Geometry: final body of the model. Coordinates: model frame, mm. A direction names the side the tool comes from. Round coordinates to 2 decimals unless told otherwise and drop trailing zeros. Return JSON: item names as keys, results as strings. Group by question number.
1. Draft query along X for faces 1 (the face through (15, 20, 13.994)), 2 (the face through (22, 29, 11.613)), 3 (the face through (24.072, 37.706, 11.299)). Return one class per face: +X half, -X half, draft (parallel to the pull), parting line (faces both ways), or undercut.
2. Material intervals for probe 1 along Y at (x, z) = (18, 12); probe 2 along Y at (x, z) = (18.5, 12); probe 3 along Z at (x, y) = (14.5, 37), sorted ascending.
3. First-contact query: pin 1 Ø1.5 at (y, z) = (7.5, 11.5) entering from +X; pin 2 Ø3 at (x, z) = (26.5, 13) entering from -Y; pin 3 Ø5 at (y, z) = (15.5, 12.5) entering from -X. Flat tips, straight axial feed; report the tip coordinate or a pass-through.
4. Set-up query: faces 4 (the face through (18, 0, 11)), 5 (the face through (11.883, 10.519, 12.82)), 6 (the face through (25.615, 17.844, 7.981)). Return all of +Z, -Z, +X, -X, +Y, -Y with unobstructed straight access to the full face (end or side cutting, diameter ignored); none if empty.
from build123d import *

# Parameters (mm, degrees)
F1_ANGLE = 18.5
F2_R     = 7.9375
F3_DEPTH = 2.38125


with BuildPart() as f1:
    # F0 (on Front) → F1 (revolve)
    with BuildSketch(Plane.XZ):
        with BuildLine():
            Line((24.2297330525, 13.9939050769), (8.419544983, 13.9939050769))
            add(Edge.make_bspline(
                [(8.419544983, 13.9939050769), (8.3193296588, 12.729684062), (9.3964822164, 9.926852923), (14.9424578975, 8.5146570379), (21.1633145653, 6.8517774271), (23.2589200169, 4.9192732328), (24.1671312945, 4.0402704404)],
                knots=[0.4603012927, 0.4603012927, 0.4603012927, 0.4603012927, 0.5552126989, 0.6720441254, 0.8004871988, 0.8904119657, 0.8904119657, 0.8904119657, 0.8904119657], degree=3))
            Line((24.1671312945, 4.0402704404), (24.2297330525, 13.9939050769))
        make_face()
    revolve(axis=Axis((136.7642762608, 0, 8.3261267356), (0, 0, -1)), revolution_arc=F1_ANGLE)

    # F2 (on face) → F3 (cut)
    with BuildSketch(Plane.XY.offset(13.9939050769)):
        with Locations((22.9123420723, 28.597757378)):
            Circle(F2_R)
        with Locations((19.7691471926, 9.6189003033)):
            Circle(F2_R)
    extrude(amount=-F3_DEPTH, mode=Mode.SUBTRACT)


solid = f1.part
Taken from the geometry:
{
 "1": {"face 1": "draft", "face 2": "undercut", "face 3": "+X half"},
 "2": {"probe 1": "0 to 1.88, 17.36 to 22.36, 34.83 to 39.74", "probe 2": "0 to 1.78, 17.45 to 22, 35.2 to 39.57", "probe 3": "11.49 to 13.99"},
 "3": {"pin 1": "x = 24.52", "pin 2": "y = 15.33", "pin 3": "x = 9.09"},
 "4": {"face 4": "+Z, -Z, +X, -X, -Y", "face 5": "+Z", "face 6": "-Z, +X, -Y"}
}
